```python
from build123d import *

# Parameters (mm, degrees)
SKETCH_W        = 70
SKETCH_H        = 120
PAD_DEPTH       = 38
SKETCH001_W     = 67.6
SKETCH001_H     = 117.6
POCKET_DEPTH    = 36.6
SKETCH112_R     = 3
PAD080_DEPTH    = 2.4
SKETCH113_R     = 1.1
POCKET031_DEPTH = 3
SKETCH136_R     = 3.5
PAD096_DEPTH    = 2.5
SKETCH137_R     = 1
POCKET039_DEPTH = 3
SKETCH138_W     = 9.2
SKETCH138_H     = 3.4
POCKET040_DEPTH = 1.401


with BuildPart() as part:
    # Sketch → Pad (new body)
    with BuildSketch(Plane.XY):
        Rectangle(SKETCH_W, SKETCH_H)
    extrude(amount=PAD_DEPTH)

    # Sketch001 (on DatumPlane) → Pocket (cut)
    with BuildSketch(Plane.XY.offset(38)):
        Rectangle(SKETCH001_W, SKETCH001_H)
    extrude(amount=-POCKET_DEPTH, mode=Mode.SUBTRACT)

    # Sketch112 → Pad080 (join)
    with BuildSketch(Plane.XY.offset(1.4)):
        with Locations((22.4, 39.500007)):
            Circle(SKETCH112_R)
        with Locations((-22.4, 39.500007)):
            Circle(SKETCH112_R)
        with Locations((-22.4, -25.499993)):
            Circle(SKETCH112_R)
        with Locations((22.4, -25.499993)):
            Circle(SKETCH112_R)
    extrude(amount=PAD080_DEPTH)

    # Sketch113 (on Face4 of Pad080) → Pocket031 (cut)
    with BuildSketch(Plane(origin=(0, 0, 0), x_dir=(1, 0, 0), z_dir=(0, 0, -1))):
        with Locations((22.4, -39.500007)):
            Circle(SKETCH113_R)
        with Locations((-22.4, -39.500007)):
            Circle(SKETCH113_R)
        with Locations((22.4, 25.499993)):
            Circle(SKETCH113_R)
        with Locations((-22.4, 25.499993)):
            Circle(SKETCH113_R)
    extrude(amount=-POCKET031_DEPTH, mode=Mode.SUBTRACT)

    # Sketch136 (on Face11 of Pad080) → Pad096 (join)
    with BuildSketch(Plane.XY.offset(1.4)):
        with Locations((20.403804, -13.646444)):
            Circle(SKETCH136_R)
        with Locations((-16.012195, -10.464463)):
            Circle(SKETCH136_R)
        with Locations((3.786795, -30.263453)):
            Circle(SKETCH136_R)
        with Locations((-8.901281, 43.65864)):
            Circle(SKETCH136_R)
        with Locations((7.715729, 27.041631)):
            Circle(SKETCH136_R)
        with Locations((-12.083261, 7.242641)):
            Circle(SKETCH136_R)
    extrude(amount=PAD096_DEPTH)

    # Sketch137 (on Face37 of Pad096) → Pocket039 (cut)
    with BuildSketch(Plane.XY.offset(3.9)):
        with Locations((-8.901281, 43.65864)):
            Circle(SKETCH137_R)
        with Locations((7.715729, 27.041631)):
            Circle(SKETCH137_R)
        with Locations((-12.083261, 7.242641)):
            Circle(SKETCH137_R)
        with Locations((-16.012195, -10.464463)):
            Circle(SKETCH137_R)
        with Locations((20.403804, -13.646444)):
            Circle(SKETCH137_R)
        with Locations((3.786795, -30.263453)):
            Circle(SKETCH137_R)
    extrude(amount=-POCKET039_DEPTH, mode=Mode.SUBTRACT)

    # Sketch138 (on Face19 of Pocket039) → Pocket040 (cut, through all)
    with BuildSketch(Plane.XY.offset(1.4)):
        with Locations((2.1, 44.7)):
            Rectangle(SKETCH138_W, SKETCH138_H)
        with Locations((-23.6, -37.7)):
            Rectangle(SKETCH138_W, SKETCH138_H)
    extrude(amount=-POCKET040_DEPTH, mode=Mode.SUBTRACT)


with BuildPart() as part_1:
    # Body placement: moved
    add(part.part.moved(Location((0, 5, 0))))


solid = part_1.part
```
For this review, take the finished solid that the model builds, in its own axes (mm). A direction names the side the tool comes from. Round coordinates to 2 decimals unless told otherwise and drop trailing zeros. Write each loop counter-clockwise with the first axis right and the second up, starting at its lowest first coordinate (ties: lowest second). Pieces come first, ordered by that corner, then holes. Notation, with made-up numbers: (53, 64) - (78, 64) arc R31 cw to (78, 102) - close; hole circle Ø11 at (82, 43). An arc over 180 degrees is marked (long way). Answer as a JSON object with one key per item and string values.
1. To check wall thickness, follow line 1 along Y through (x, z) = (-22.4, 1); line 2 along Y through (x, z) = (-22.4, 1.75); line 3 along X through (y, z) = (-44, 2.5). State the ranges of each line that lie inside material, in increasing order.
Response values:
{"line 1": "y = -55 to -34.4, -31 to -21.6, -19.4 to 43.4, 45.6 to 65", "line 2": "y = -55 to -53.8, -23.5 to -21.6, -19.4 to -17.5, 41.5 to 43.4, 45.6 to 47.5, 63.8 to 65", "line 3": "x = -35 to -33.8, 33.8 to 35"}
2. Tool access review of faces 1 (the face through (-33.8, 4, 20)), 2 (the face through (0, -55, 19)), 3 (the face through (22.99, -21.43, 1.48)): name each direction out of +Z, -Z, +X, -X, +Y, -Y from which nothing blocks a thin tool from reaching the whole face with its end or side.
Response values:
{"face 1": "+Z", "face 2": "+Z, -Z, +X, -X, -Y", "face 3": "-Z"}
3. We need section A-A on y = 7. Give the boundary of the cut face in (x, z).
Response values:
{"outline": "(-35, 0) - (35, 0) - (35, 38) - (33.8, 38) - (33.8, 1.4) - (-33.8, 1.4) - (-33.8, 38) - (-35, 38) - close"}
4. Draft analysis for pull direction X (two halves, no side actions). For faces 4 (the face through (0, 65, 19)), 5 (the face through (35, 4, 19)), 6 (the face through (-14.66, 14.61, 2.63)), state which applies: +X half, -X half, draft (parallel to the pull), parting line (faces both ways), or undercut.
Response values:
{"face 4": "draft", "face 5": "+X half", "face 6": "undercut"}
5. For pin 1 Ø0.7 at (x, y) = (22.5, 45) entering from -Z; pin 2 Ø0.6 at (x, y) = (4, -25) entering from +Z; pin 3 Ø7.5 at (x, y) = (-13.5, 13.5) entering from +Z, all flat-tipped, find the tip position at first contact; note any pin that passes through.
Response values:
{"pin 1": "stops at z = 3", "pin 2": "stops at z = 0.9", "pin 3": "stops at z = 3.9"}
6. We need section B-B on z = 20.5. Give the boundary of the cut face in (x, y), then the cut area to 3 significant figures.
Response values:
{"outline": "(-35, -55) - (35, -55) - (35, 65) - (-35, 65) - close; hole (-33.8, -53.8) - (33.8, -53.8) - (33.8, 63.8) - (-33.8, 63.8) - close", "area": "450 mm2"}
7. We need section C-C on x = 13. Give the boundary of the cut face in (y, z).
Response values:
{"outline": "(-55, 0) - (65, 0) - (65, 38) - (63.8, 38) - (63.8, 1.4) - (-53.8, 1.4) - (-53.8, 38) - (-55, 38) - close"}
